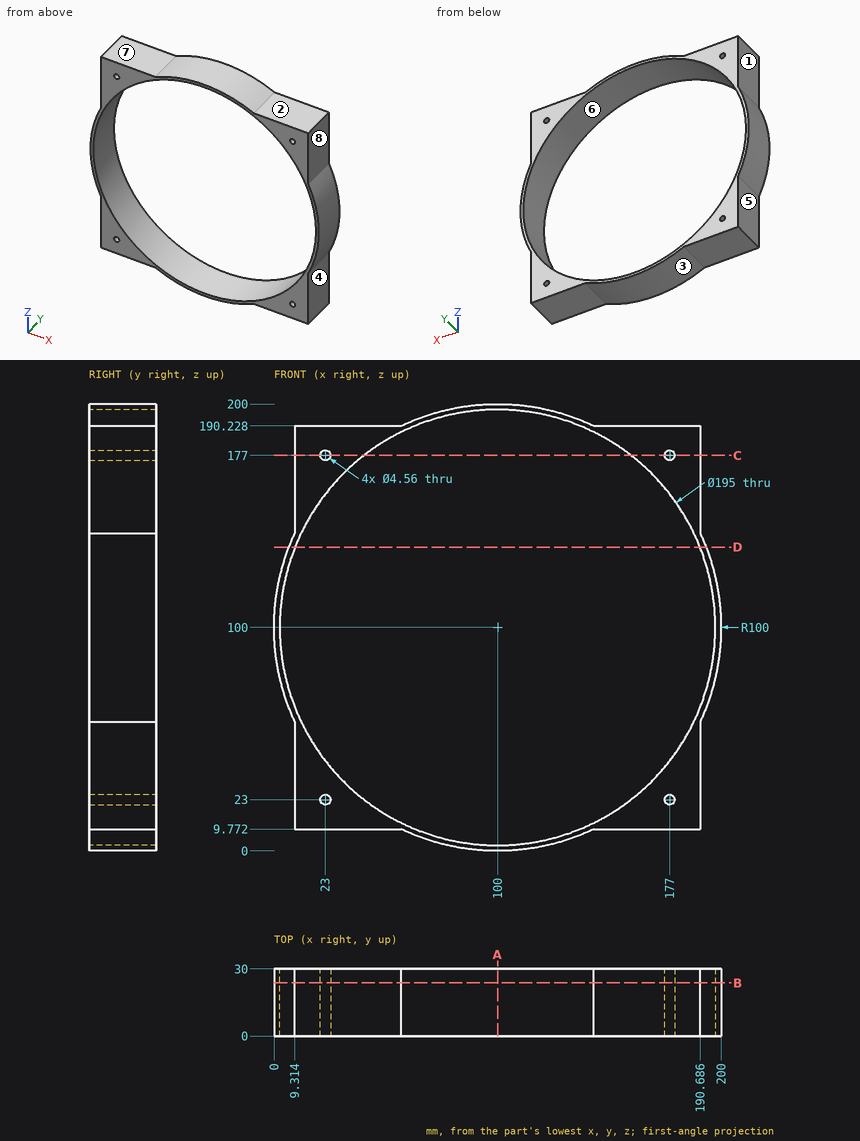
Geometry check sheet. Reference: drawing and pictorial views, mm from the part's lowest x, y, z. A direction names the side the tool comes from. Give positions to 0.01 mm unless a question says otherwise; leave off trailing zeros. Order: outer loops, then holes, each group sorted by start corner. A loop starts at its lowest first (then second) coordinate and runs counter-clockwise, first axis right, second up. Notation, with made-up numbers: M 28.25,80 L 51.25,80 A16 ccw 51.25,96 Z; hole C 56.25,67.25 d7. An arc over 180 degrees is marked long. Answer as CSV lines item,"result". Start each with the question number.
Item 1: Cross-section at C-C on z = 177. Enter the section's corners in (x, y), plus the area to 3 significant figures.
Item 2: Gauge pin test, flat ends, axial feed: P1, Ø12, axis at y = 12, z = 151.5, coming from the -X side; P2, Ø15, axis at x = 24, y = 18, coming from the +Z side; P3, Ø9, axis at x = 165.5, y = 10.5, coming from the -Z side; P4, Ø3.5, axis at x = 23, z = 177, coming from the +Y side (3 decimals). Record the tip position at first contact, or that the pin passes through.
Item 3: Mould release check, pull along Z, two halves, no side actions. Record for the marked faces 6, 7 and 8: +Z half, -Z half, draft (parallel to the pull), parting line (faces both ways), or undercut.
Item 4: Cross-section at D-D on z = 136. Enter the section's corners in (x, y) (1 decimal), plus the area to 3 significant figures.
Item 5: Cross-section at B-B on y = 23.75. Enter the section's corners in (x, z).
Item 6: Thickness scan on line 1 (Z direction, x = 100, y = 12.25); line 2 (Z direction, x = 177, y = 22.25). Record the ranges inside material, lowest first. Write a range as [from, to].
Item 7: Tool access check on the marked faces 1, 2, 3, 4 and 5. Record the directions out of +Z, -Z, +X, -X, +Y, -Y that give a thin tool (end or side, any length) a straight path to the whole face; none if there is none.
Item 8: Cross-section at A-A on x = 100. Enter the section's corners in (y, z).
Established:
1,outline,"M 9.31,0 L 20.72,0 L 20.72,30 L 9.31,30 Z; M 25.28,0 L 40.19,0 L 40.19,30 L 25.28,30 Z; M 159.81,0 L 174.72,0 L 174.72,30 L 159.81,30 Z; M 179.28,0 L 190.69,0 L 190.69,30 L 179.28,30 Z"
1,area,"1,580 mm^2"
2,P1,"stops at x = 9.31"
2,P2,"stops at z = 190.23"
2,P3,"stops at z = 9.77"
2,P4,"passes through"
3,face 6,"undercut"
3,face 7,"+Z half"
3,face 8,"draft"
4,outline,"M 6.7,0 L 9.4,0 L 9.4,30 L 6.7,30 Z; M 190.6,0 L 193.3,0 L 193.3,30 L 190.6,30 Z"
4,area,"161 mm^2"
5,outline,"M 9.31,9.77 L 56.88,9.77 A100 ccw 143.12,9.77 L 190.69,9.77 L 190.69,57.86 A100 ccw 190.69,142.14 L 190.69,190.23 L 143.12,190.23 A100 ccw 56.88,190.23 L 9.31,190.23 L 9.31,142.14 A100 ccw 9.31,57.86 Z; hole C 100,100 d195; hole C 23,23 d4.56; hole C 23,177 d4.56; hole C 177,23 d4.56; hole C 177,177 d4.56"
6,line 1,"z = [0, 2.5], [197.5, 200]"
6,line 2,"z = [9.77, 20.72], [25.28, 40.19], [159.81, 174.72], [179.28, 190.23]"
7,face 1,"+Z, -X, +Y, -Y"
7,face 2,"+Z, +X, +Y, -Y"
7,face 3,"-Z, +Y, -Y"
7,face 4,"-Z, +X, +Y, -Y"
7,face 5,"-Z, -X, +Y, -Y"
8,outline,"M 0,0 L 30,0 L 30,2.5 L 0,2.5 Z; M 0,197.5 L 30,197.5 L 30,200 L 0,200 Z"
